```python
from build123d import *

# Parameters (mm, degrees)
SKETCH1_R               = 4
SKETCH1_R_2             = 0.75
BOSS_EXTRUDE1_DEPTH     = 5
SKETCH2_W               = 7
SKETCH2_H               = 2.5
CUT_EXTRUDE1_DEPTH      = 5
CUT_EXTRUDE1_DEPTH_BACK = 5


with BuildPart() as part:
    # Sketch1 → Boss-Extrude1 (new body)
    with BuildSketch(Plane.XY):
        Polygon((-30.771428571, -18.807142857), (-4.771428571, -18.807142857), (2.228571429, -10.807142857), (2.228571429, -6.807142857), (-4.771428571, 1.192857143), (-30.771428571, 1.192857143), (-37.771428571, -6.807142857), (-37.771428571, -10.807142857), align=None)
        with Locations((-17.771428571, -8.807142857)):
            Circle(SKETCH1_R, mode=Mode.SUBTRACT)
        with Locations((-17.629745485, -2.058630135)):
            Circle(SKETCH1_R_2, mode=Mode.SUBTRACT)
        with Locations((-17.913111664, -15.555655867)):
            Circle(SKETCH1_R_2, mode=Mode.SUBTRACT)
    extrude(amount=BOSS_EXTRUDE1_DEPTH)

    # Sketch2 → Cut-Extrude1 (cut, two sides)
    with BuildSketch(Plane.XY.offset(5)) as cut_extrude1_sk:
        with Locations((-29.271428571, -7.557142857)):
            Rectangle(SKETCH2_W, SKETCH2_H)
        with Locations((-29.271428571, -10.057142857)):
            Rectangle(SKETCH2_W, SKETCH2_H)
        with Locations((-6.271428571, -7.557142857)):
            Rectangle(SKETCH2_W, SKETCH2_H)
        with Locations((-6.271428571, -10.057142857)):
            Rectangle(SKETCH2_W, SKETCH2_H)
    extrude(amount=CUT_EXTRUDE1_DEPTH, mode=Mode.SUBTRACT)
    extrude(cut_extrude1_sk.sketch, amount=-CUT_EXTRUDE1_DEPTH_BACK, mode=Mode.SUBTRACT)


solid = part.part
```
Source: CAD feature listing. Evaluate the final solid. Frame: model axes, mm. A direction names the side the tool comes from. Give positions to 0.01 mm unless a question says otherwise; leave off trailing zeros. Loops run counter-clockwise (first coordinate to the right, second up) from the corner with the lowest first, then second, coordinate; pieces in that order, holes last. Notation, with made-up numbers: (11, -27) -> (35, -27) arc R25 ccw to (35, -8) -> close; hole circle Ø10 at (-2.5, 59.5). An arc over 180 degrees is marked (long way). Put each result on its own line as item: value. Start each with the question number.
1) Reachability of faces 1 (the face through (-1.32, -14.86, 2.46)), 2 (the face through (-9.771, -9, 3)) from +Z, -Z, +X, -X, +Y, -Y: full face, straight path, thin tool, end or side. Return the list, or none.
2) Cut plane A-A (y = -5.5). Return loops of the section in (x, z).
3) Material intervals for probe 1 along X at (y, z) = (-9, 0.75); probe 2 along Y at (x, z) = (-7, 3.8); probe 3 along X at (y, z) = (-9.25, 3.2), sorted ascending.
4) Cut plane C-C (x = -15). Return loops of the section in (y, z).
5) Cut plane B-B (z = 3.3). Return loops of the section in (x, y).
6) Cut plane D-D (y = -7.5). Return loops of the section in (x, z), then the cut area to 3 significant figures.
7) Draft query along X for faces 3 (the face through (-13.6, -8.7, 5)), 4 (the face through (-34.22, -2.75, 2.46)), 5 (the face through (-13.956, -7.606, 2.465)). Return one class per face: released by +X, released by -X, zero draft, split by the parting line, or undercut.
8) Contact query for flat-ended pins moving along their axis: P1, Ø3, axis at x = -27.5, y = -8.5, coming from the -Z side; P2, Ø2, axis at y = -4, z = 2.5, coming from the +X side; P3, Ø3, axis at y = -13.5, z = 4.5, coming from the +X side. Output: stop coordinate, or through.
Results are:
1. face 1: +Z, -Z, +X, -Y
1. face 2: +Z, -Z
2. outline: (-36.63, 0) -> (-20.02, 0) -> (-20.02, 5) -> (-36.63, 5) -> close; (-15.52, 0) -> (1.08, 0) -> (1.08, 5) -> (-15.52, 5) -> close
3. probe 1: x = -37.77 to -32.77, -25.77 to -21.77, -13.78 to -9.77, -2.77 to 2.23
3. probe 2: y = -18.81 to -11.31, -6.31 to 1.19
3. probe 3: x = -37.77 to -32.77, -25.77 to -21.75, -13.8 to -9.77, -2.77 to 2.23
4. outline: (-18.81, 0) -> (-11.69, 0) -> (-11.69, 5) -> (-18.81, 5) -> close; (-5.92, 0) -> (1.19, 0) -> (1.19, 5) -> (-5.92, 5) -> close
5. outline: (-37.77, -10.81) -> (-30.77, -18.81) -> (-4.77, -18.81) -> (2.23, -10.81) -> (2.23, -6.81) -> (-4.77, 1.19) -> (-30.77, 1.19) -> (-37.77, -6.81) -> close; hole (-32.77, -11.31) -> (-25.77, -11.31) -> (-25.77, -6.31) -> (-32.77, -6.31) -> close; hole circle Ø8 at (-17.77, -8.81); hole circle Ø1.5 at (-17.91, -15.56); hole circle Ø1.5 at (-17.63, -2.06); hole (-9.77, -11.31) -> (-2.77, -11.31) -> (-2.77, -6.31) -> (-9.77, -6.31) -> close
6. outline: (-37.77, 0) -> (-32.77, 0) -> (-32.77, 5) -> (-37.77, 5) -> close; (-25.77, 0) -> (-21.55, 0) -> (-21.55, 5) -> (-25.77, 5) -> close; (-13.99, 0) -> (-9.77, 0) -> (-9.77, 5) -> (-13.99, 5) -> close; (-2.77, 0) -> (2.23, 0) -> (2.23, 5) -> (-2.77, 5) -> close
6. area: 92.2 mm2
7. face 3: zero draft
7. face 4: released by -X
7. face 5: undercut
8. P1: passes through
8. P2: stops at x = 0.65
8. P3: stops at x = 1.18
